Autodesk Inventor part; units mm, degrees
ref_plane "YZ Plane" through (0, 0, 0) normal (1, 0, 0) x (0, 1, 0)
ref_plane "XZ Plane" through (0, 0, 0) normal (0, 1, 0) x (-1, 0, 0)
ref_plane "XY Plane" through (0, 0, 0) normal (0, 0, 1) x (1, 0, 0)
sketch "Эскиз1" plane through (0, 0, 0) normal (0, 1, 0) x (-1, 0, 0)
  line L0 (0, 0) -> (70, 0)
  line L1 (70, 0) -> (70, -100)
  line L2 (70, -100) -> (0, -100)
  line L3 (0, -100) -> (0, 0)
  dimension "d0" = 70
  dimension "d1" = 100
extrude "Выдавливание1" add sketch "Эскиз1" along normal blind 10
sketch "Эскиз2" plane through (0, 10, 0) normal (0, 1, 0) x (1, 0, 0)
  line L0 (0, 0) -> (0, 100)
  line L1 (0, 50) -> (-45, 50)
  circle A0 centre (-45, 50) radius 5
  line L2 (0, 50) -> (0, 65)
  line L3 (0, 65) -> (-45, 65)
  line L4 (0, 50) -> (0, 35)
  line L5 (0, 35) -> (-45, 35)
  line L6 (-45, 50) -> (-70, 50)
  line L7 (-70, 100) -> (-70, 0)
  line L8 (-45, 50) -> (5, 50) construction
  line L9 (-45, 50) -> (-52.1103, 25.1139)
  line L10 (-45, 50) -> (15, 50) construction
  line L11 (-45, 50) -> (-52.1103, 74.8861)
  circle A1 centre (-45, 50) radius 9
  line L12 (-45, 65) -> (-55, 100)
  line L13 (-45, 35) -> (-55, 0)
  line L14 (-55, 0) -> (0, 0)
  line L15 (0, 0) -> (0, 100)
  line L16 (0, 100) -> (-55, 100)
  dimension "d4" = 45
  dimension "d5" = 10
  dimension "d6" = 15
  dimension "d7" = 15
  dimension "d13" = 18
  dimension "d19" = 45
  dimension "d49" = 55
  dimension "d50" = 148.109
extrude "Выдавливание2" add sketch "Эскиз2" along normal blind 10 contours L14 L13 L5 L0 | L3 L12 L16 L0
extrude "Выдавливание3" cut sketch "Эскиз2" against normal blind 42.5 contours A0 L9 L1 | L1 L11 A0 | L9 A0 L6 | L6 A0 L11
sketch "Эскиз3" plane through (0, 0, 0) normal (0, -1, 0) x (1, 0, 0)
  circle A0 centre (-45, -50) radius 5
  line L0 (-45, -50) -> (-15, -50)
  circle A1 centre (-15, -50) radius 6
  point P0 (0, 0)
  dimension "d20" = 30
  dimension "d21" = 12
extrude "Выдавливание4" cut sketch "Эскиз3" against normal blind 3 contours A1
chamfer "Фаска1" distance 1 angle 45 1 edges at (-21, 0, -50)
sketch "Эскиз4" plane through (0, 0, 0) normal (1, 0, 0) x (0, 0, -1)
  line L0 (0, 0) -> (0, 20)
  line L1 (0, 0) -> (-15, 0)
  line L2 (-15, 0) -> (-15, 20)
  line L3 (-15, 20) -> (0, 20)
  line L4 (0, 20) -> (0, 0)
  line L5 (100, 0) -> (100, 20)
  line L6 (100, 0) -> (115, 0)
  line L7 (115, 0) -> (115, 20)
  line L8 (115, 20) -> (100, 20)
  line L9 (100, 20) -> (100, 0)
  line L10 (115, 20) -> (110, 20)
  line L11 (110, 20) -> (110, 10)
  line L12 (110, 10) -> (115, 10)
  line L13 (115, 10) -> (115, 20)
  line L14 (-15, 20) -> (-10, 20)
  line L15 (-10, 20) -> (-10, 10)
  line L16 (-10, 10) -> (-15, 10)
  line L17 (-15, 10) -> (-15, 20)
  circle A0 centre (-10, 10) radius 3
  circle A1 centre (110, 10) radius 3
  line L18 (100, 20) -> (0, 20)
  dimension "d27" = 15
  dimension "d28" = 15
  dimension "d29" = 5
  dimension "d30" = 10
  dimension "d31" = 5
  dimension "d32" = 10
  dimension "d33" = 6
  dimension "d34" = 6
extrude "Выдавливание5" add sketch "Эскиз4" against normal blind 3 contours L1 L2 L16 A0 L15 L3 L0 | L8 L11 A1 L12 L7 L6 L5 | L15 A0 L16 L2 L3 | L8 L7 L12 A1 L11
properties part number "Стенка"
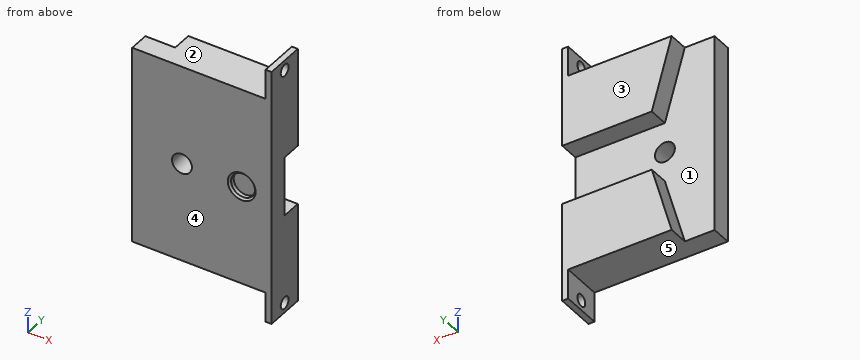
Work out the finished part from the listing and answer in its coordinate system (mm). Face numbers are marked on the shaded views. A direction names the side the tool comes from. Round coordinates to 2 decimals unless told otherwise and drop trailing zeros. Write each loop counter-clockwise with the first axis right and the second up, starting at its lowest first coordinate (ties: lowest second). Pieces come first, ordered by that corner, then holes. Notation, with made-up numbers: (11, -18) - (37, -18) arc R25 cw to (37, 2) - close; hole circle Ø3 at (14.5, 89). An arc over 180 degrees is marked (long way). Answer in a Markdown table with one row per item. Add a question column.
1. A cutting plane is placed at A-A, the plane z = -110. Determine the outline of the cut face in (x, y), and give its area (3 significant figures).
2. A cutting plane is placed at B-B, the plane y = 15.5. Determine the outline of the cut face in (x, z).
3. Find the intervals of material crossed by line 1 along X through (y, z) = (2.35, -50); line 2 along Z through (x, y) = (-13, 16); line 3 along Z through (x, y) = (-45, 2.75), in increasing order. Write a range as from..to.
4. Given pin 1 (4 mm diameter, centred on x = -13.5, y = 9, fed in from -Z); pin 2 (12 mm diameter, centred on x = -25.5, z = -54, fed in from +Y); pin 3 (5.5 mm diameter, centred on y = 10, z = 10, fed in from -X); pin 4 (9.5 mm diameter, centred on x = -15, z = -50, fed in from -Y), each flat-ended and moving along its own axis, determine where each tip first touches the part or whether it passes through.
5. A cutting plane is placed at C-C, the plane x = -42.5. Determine the outline of the cut face in (y, z), and give its area (3 significant figures).
6. A cutting plane is placed at D-D, the plane z = -50. Determine the outline of the cut face in (x, y), and give its area (3 significant figures).
7. The mould has two halves that part along Z. Classify the marked faces 1, 2 and 3: +Z half, -Z half, draft (parallel to the pull), parting line (faces both ways), or undercut.
8. For the marked faces 4 and 5, determine the directions among +Z, -Z, +X, -X, +Y, -Y from which every point of the face is accessible in a straight line to the end or side of a thin tool.
Worked out:
| question | item | result |
|---|---|---|
| 1 | outline | (-3, 0) - (0, 0) - (0, 7) - (-3, 7) - close; (-3, 13) - (0, 13) - (0, 20) - (-3, 20) - close |
| 1 | area | 42.0 mm^2 |
| 2 | outline | (-55, -100) - (-3, -100) - (-3, -115) - (0, -115) - (0, -65) - (-45, -65) - close; (-55, 0) - (-45, -35) - (0, -35) - (0, 15) - (-3, 15) - (-3, 0) - close |
| 3 | line 1 | -70..-50, -40..-21, -9..0 |
| 3 | line 2 | -100..-65, -35..0 |
| 3 | line 3 | -100..-55, -45..0 |
| 4 | pin 1 | z = -100 |
| 4 | pin 2 | y = 10 |
| 4 | pin 3 | through |
| 4 | pin 4 | y = 3 |
| 5 | outline | (0, -100) - (20, -100) - (20, -65) - (10, -65) - (10, -54.33) - (0, -54.33) - close; (0, -45.67) - (10, -45.67) - (10, -35) - (20, -35) - (20, 0) - (0, 0) - close |
| 5 | area | 1,610 mm^2 |
| 6 | outline | (-70, 0) - (-50, 0) - (-50, 10) - (-70, 10) - close; (-40, 0) - (-22, 0) - (-21, 1) - (-21, 3) - (-9, 3) - (-9, 1) - (-8, 0) - (0, 0) - (0, 10) - (-40, 10) - close |
| 6 | area | 563 mm^2 |
| 7 | face 1 | undercut |
| 7 | face 2 | +Z half |
| 7 | face 3 | draft |
| 8 | face 4 | +Z, -Z, +X, -X, -Y |
| 8 | face 5 | -Z, -X, +Y, -Y |
